Geometry: final body of the model. Coordinates: model frame, mm. Face numbers are marked on the shaded views. A direction names the side the tool comes from. Round coordinates to 2 decimals unless told otherwise and drop trailing zeros. Order: outer loops, then holes, each group sorted by start corner. A loop starts at its lowest first (then second) coordinate and runs counter-clockwise, first axis right, second up. Notation, with made-up numbers: (55.5, -39) - (78.5, -39) arc R9 ccw to (78.5, -25) - close; hole circle Ø1 at (-5, 9). An arc over 180 degrees is marked (long way). Put each result on its own line as item: value. Start each with the question number.
(1) Section A-A (y = -0.5). Output: boundary loops of the cut face in (x, z).
(2) Material intervals for L1, parallel to Y at x = -22.75, z = 5; L2, parallel to Z at x = -22, y = -9.25; L3, parallel to Y at x = -14.25, z = 11.75, sorted ascending. Write a range as [from, to].
(3) Pull-direction query (Y, two-part tool) for the marked faces 1, 2 and 3; classes: released by +Y, released by -Y, zero draft, split by the parting line, or undercut.
(4) Section D-D (y = -8). Count the separate pieces of the cut face and the enclosed holes in it, and give its area (3 significant figures).
(5) Access query for the marked faces 4 and 5. Directions: +Z, -Z, +X, -X, +Y, -Y. A direction counts if a zero-diameter tool reaches every point of the face in a straight line with its end or side. Return the directions, or none.
(6) Section B-B (z = 10). Output: boundary loops of the cut face in (x, y).
(7) Pin query (flat end, axial travel): P1, Ø1.5, axis at y = -4.5, z = 3.5, coming from the +X side; P2, Ø0.7, axis at y = 3.5, z = 17, coming from the +X side; P3, Ø1, axis at x = -10, z = 13.5, coming from the -Y side; P4, Ø3.5, axis at y = -7.99, z = 15, coming from the +X side. Return the tip coordinate at first contact, or that it passes through.
(8) Section C-C (x = -6.75). Output: boundary loops of the cut face in (y, z).
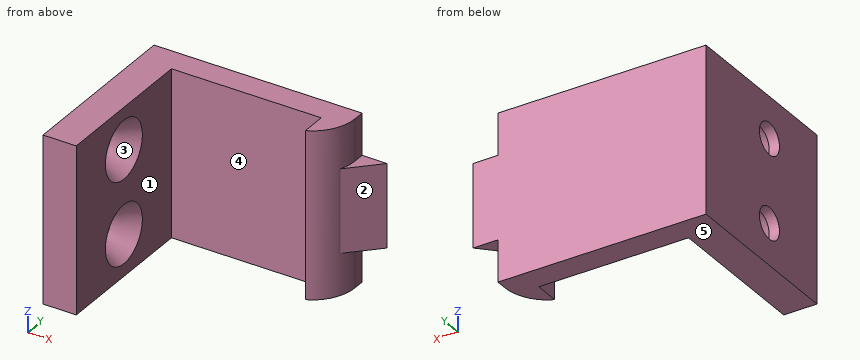
from build123d import *

# Parameters (mm, degrees)
F1_DEPTH       = 20
F2_DEPTH       = 15
F3_DEPTH       = 5
F5_D           = 3.8
F5_DEPTH       = 20
F5_CSINK_D     = 7
F5_CSINK_ANGLE = 60
F5_TIP         = 1.1416351762
F6_T4_DEPTH    = 43.1732604525
F6_T10_DEPTH   = 43.1732604525
F6_T16_DEPTH   = 43.1732604525
F6_T23_DEPTH   = 43.1732604525
F6_T29_DEPTH   = 43.1732604525


# Not quite as in the source:
# - a fillet or chamfer that OpenCascade refuses, or shapes differently, is made with other operations: its cross-section is extruded or revolved along the edge and cut away or added


with BuildPart() as f1:
    # F0 (on Top) → F1 (new body)
    with BuildSketch(Plane.XY):
        Polygon((-23.1947004795, 4.0139819533), (-23.1947004795, -16.9860180467), (-19.1947004795, -16.9860180467), (-19.1947004795, 1.0139819533), (-1.1947004795, 1.0139819533), (-1.1947004795, -1.9860180467), (1.8052995205, -1.9860180467), (1.8052995205, 1.0139819533), (1.8052995205, 4.0139819533), align=None)
    extrude(amount=F1_DEPTH)

    # F0 (on Top) → F2 (join)
    with BuildSketch(Plane.XY):
        Polygon((4.8052995205, 4.0139819533), (1.8052995205, 4.0139819533), (1.8052995205, 1.0139819533), align=None)
    extrude(amount=F2_DEPTH)

    # F0 (on Top) → F3 (cut)
    with BuildSketch(Plane.XY):
        Polygon((4.8052995205, 4.0139819533), (1.8052995205, 4.0139819533), (1.8052995205, 1.0139819533), align=None)
    extrude(amount=F3_DEPTH, mode=Mode.SUBTRACT)

    # F5
    with Locations(Plane.YZ.offset(-19.1947004795)):
        with Locations((-7.9860180467, 15), (-7.9860180467, 5)):
            CounterSinkHole(F5_D / 2, F5_CSINK_D / 2, depth=F5_DEPTH, counter_sink_angle=F5_CSINK_ANGLE)
            with Locations((0, 0, -(F5_DEPTH + F5_TIP / 2))):  # 118° drill point
                Cone(0, F5_D / 2, F5_TIP, mode=Mode.SUBTRACT)

    # F6: fillet of radius 5.08 on 1 edges, made by hand


with BuildPart() as f6_tool2:
    # F6_s3 → F6_t4 (new body)
    with BuildSketch(Plane.XY.offset(-11.5866302263)):
        with BuildLine():
            ThreePointArc((1.8052995205, 2.6486340438), (0.9898510796, -0.1118007046), (-1.1947004795, -1.9860180467))
            Line((-1.1947004795, -1.9860180467), (-1.1531004795, -2.0787110885))
            ThreePointArc((-1.1531004795, -2.0787110885), (0.3052995205, -2.0876180467), (1.8052995205, -2.0876180467))
            Line((1.8052995205, -2.0876180467), (1.9068995205, -1.9860180467))
            Line((1.9068995205, -1.9860180467), (1.9068995205, 2.6486340438))
            Line((1.9068995205, 2.6486340438), (1.8052995205, 2.6486340438))
        make_face()
    extrude(amount=F6_T4_DEPTH)

    split(bisect_by=Plane(origin=(0.3956587836, -0.3956587836, 0), x_dir=(0, 0, 1), z_dir=(-0.7071067812, 0.7071067812, 0)), keep=Keep.TOP)

    split(bisect_by=Plane.XY.offset(5), keep=Keep.BOTTOM)


with BuildPart() as f1_1:
    add(f1.part)

    # F6_t1: cut F6_tool2
    add(f6_tool2.part, mode=Mode.SUBTRACT)


with BuildPart() as f6_tool8:
    # F6_s9 → F6_t10 (new body)
    with BuildSketch(Plane.XY.offset(-11.5866302263)):
        with BuildLine():
            ThreePointArc((1.8052995205, 2.6486340438), (0.9898510796, -0.1118007046), (-1.1947004795, -1.9860180467))
            Line((-1.1947004795, -1.9860180467), (-1.1531004795, -2.0787110885))
            ThreePointArc((-1.1531004795, -2.0787110885), (0.3052995205, -2.0876180467), (1.8052995205, -2.0876180467))
            Line((1.8052995205, -2.0876180467), (1.9068995205, -1.9860180467))
            Line((1.9068995205, -1.9860180467), (1.9068995205, 2.6486340438))
            Line((1.9068995205, 2.6486340438), (1.8052995205, 2.6486340438))
        make_face()
    extrude(amount=F6_T10_DEPTH)

    split(bisect_by=Plane(origin=(0.3956587836, -0.3956587836, 0), x_dir=(0, 0, 1), z_dir=(0.7071067812, -0.7071067812, 0)), keep=Keep.TOP)

    split(bisect_by=Plane.XY.offset(5), keep=Keep.BOTTOM)


with BuildPart() as f1_2:
    add(f1_1.part)

    # F6_t7: cut F6_tool8
    add(f6_tool8.part, mode=Mode.SUBTRACT)


with BuildPart() as f6_tool14:
    # F6_s15 → F6_t16 (new body)
    with BuildSketch(Plane.XY.offset(-11.5866302263)):
        with BuildLine():
            ThreePointArc((1.8052995205, 2.6486340438), (0.9898510796, -0.1118007046), (-1.1947004795, -1.9860180467))
            Line((-1.1947004795, -1.9860180467), (-1.1531004795, -2.0787110885))
            ThreePointArc((-1.1531004795, -2.0787110885), (0.3052995205, -2.0876180467), (1.8052995205, -2.0876180467))
            Line((1.8052995205, -2.0876180467), (1.9068995205, -1.9860180467))
            Line((1.9068995205, -1.9860180467), (1.9068995205, 2.6486340438))
            Line((1.9068995205, 2.6486340438), (1.8052995205, 2.6486340438))
        make_face()
    extrude(amount=F6_T16_DEPTH)

    split(bisect_by=Plane.XY.offset(15), keep=Keep.BOTTOM)

    split(bisect_by=Plane(origin=(0.3956587836, -0.3956587836, 0), x_dir=(0, 0, 1), z_dir=(0.7071067812, -0.7071067812, 0)), keep=Keep.TOP)

    split(bisect_by=Plane.XY.offset(5), keep=Keep.TOP)


with BuildPart() as f1_3:
    add(f1_2.part)

    # F6_t13: cut F6_tool14
    add(f6_tool14.part, mode=Mode.SUBTRACT)


with BuildPart() as f6_tool21:
    # F6_s22 → F6_t23 (new body)
    with BuildSketch(Plane.XY.offset(-11.5866302263)):
        with BuildLine():
            ThreePointArc((1.8052995205, 2.6486340438), (0.9898510796, -0.1118007046), (-1.1947004795, -1.9860180467))
            Line((-1.1947004795, -1.9860180467), (-1.1531004795, -2.0787110885))
            ThreePointArc((-1.1531004795, -2.0787110885), (0.3052995205, -2.0876180467), (1.8052995205, -2.0876180467))
            Line((1.8052995205, -2.0876180467), (1.9068995205, -1.9860180467))
            Line((1.9068995205, -1.9860180467), (1.9068995205, 2.6486340438))
            Line((1.9068995205, 2.6486340438), (1.8052995205, 2.6486340438))
        make_face()
    extrude(amount=F6_T23_DEPTH)

    split(bisect_by=Plane.XY.offset(15), keep=Keep.TOP)

    split(bisect_by=Plane(origin=(0.3956587836, -0.3956587836, 0), x_dir=(0, 0, 1), z_dir=(-0.7071067812, 0.7071067812, 0)), keep=Keep.TOP)


with BuildPart() as f1_4:
    add(f1_3.part)

    # F6_t20: cut F6_tool21
    add(f6_tool21.part, mode=Mode.SUBTRACT)


with BuildPart() as f6_tool27:
    # F6_s28 → F6_t29 (new body)
    with BuildSketch(Plane.XY.offset(-11.5866302263)):
        with BuildLine():
            ThreePointArc((1.8052995205, 2.6486340438), (0.9898510796, -0.1118007046), (-1.1947004795, -1.9860180467))
            Line((-1.1947004795, -1.9860180467), (-1.1531004795, -2.0787110885))
            ThreePointArc((-1.1531004795, -2.0787110885), (0.3052995205, -2.0876180467), (1.8052995205, -2.0876180467))
            Line((1.8052995205, -2.0876180467), (1.9068995205, -1.9860180467))
            Line((1.9068995205, -1.9860180467), (1.9068995205, 2.6486340438))
            Line((1.9068995205, 2.6486340438), (1.8052995205, 2.6486340438))
        make_face()
    extrude(amount=F6_T29_DEPTH)

    split(bisect_by=Plane.XY.offset(15), keep=Keep.TOP)

    split(bisect_by=Plane(origin=(0.3956587836, -0.3956587836, 0), x_dir=(0, 0, 1), z_dir=(0.7071067812, -0.7071067812, 0)), keep=Keep.TOP)


with BuildPart() as f1_5:
    add(f1_4.part)

    # F6_t26: cut F6_tool27
    add(f6_tool27.part, mode=Mode.SUBTRACT)


solid = f1_5.part
Checks:
1. outline: (-23.19, 0) - (-19.19, 0) - (-19.19, 20) - (-23.19, 20) - close; (-1.19, 0) - (0.71, 0) - (0.71, 20) - (-1.19, 20) - close
2. L1: y = [-16.99, -9.89], [-6.09, 4.01]
2. L2: z = [0, 3.58], [6.42, 13.58], [16.42, 20]
2. L3: y = [1.01, 4.01]
3. face 1: zero draft
3. face 2: released by -Y
3. face 3: undercut
4. separate pieces: 3
4. enclosed holes: 0
4. area: 40.7 mm²
5. face 4: +Z, -Z, -Y
5. face 5: -Z, +X, -X, +Y, -Y
6. outline: (-23.19, -16.99) - (-19.19, -16.99) - (-19.19, 1.01) - (-1.19, 1.01) - (-1.19, -1.99) arc R5.08 ccw to (1.36, 0.57) - (4.81, 4.01) - (-23.19, 4.01) - close
7. P1: stops at x = -19.19
7. P2: stops at x = 1.81
7. P3: stops at y = 1.01
7. P4: passes through
8. outline: (1.01, 0) - (4.01, 0) - (4.01, 20) - (1.01, 20) - close
